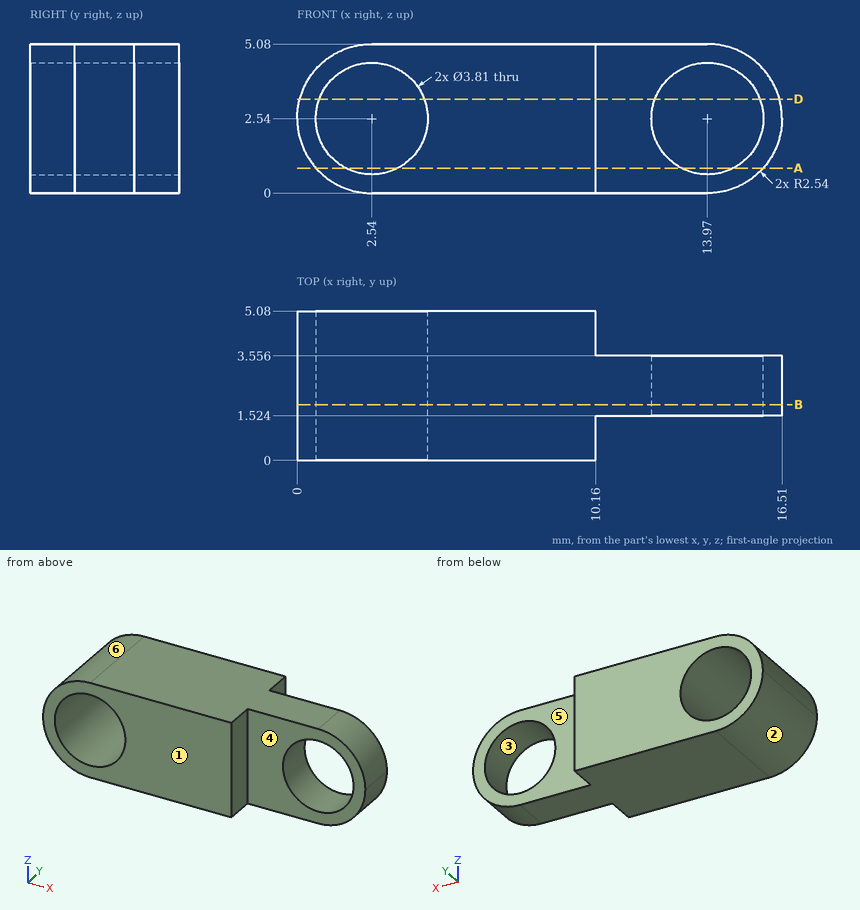
Geometry check sheet. Reference: drawing and pictorial views, mm from the part's lowest x, y, z. A direction names the side the tool comes from. Give positions to 0.01 mm unless a question says otherwise; leave off trailing zeros. Order: outer loops, then holes, each group sorted by start corner. A loop starts at its lowest first (then second) coordinate and runs counter-clockwise, first axis right, second up. Notation, with made-up numbers: M 20.25,70.25 L 62.25,70.25 A20 ccw 62.25,93.25 Z; hole C 53.25,36 d5. An arc over 180 degrees is marked long. Answer as a JSON object with one key per item and string values. Group by question number.
1) Cross-section at B-B (y = 1.9). Give the number of separate pieces and of enclosed holes in the cut face, then the cut area to 3 significant figures.
2) Depth check by flat-ended pin: pin 1 Ø0.8 at (y, z) = (0.5, 3) entering from +X; pin 2 Ø2.5 at (x, z) = (13.97, 2.54) entering from +Y; pin 3 Ø1 at (y, z) = (2, 1.5) entering from +X. Enter the tip coordinate at first touch or a pass-through.
3) Cross-section at A-A (z = 0.85). Enter the section's corners in (x, y).
4) Access from +Z, -Z, +X, -X, +Y, -Y to the whole of each face (thin tool, end or side, straight path). Record for the marked faces 4, 5 and 6.
5) Scan lines: line 1 along Z through (x, y) = (2.5, 1.8); line 2 along X through (y, z) = (2.65, 2.7); line 3 along X through (y, z) = (3.15, 1.8). Record each from-to range of solid material in increasing order. Write a range as [from, to].
6) Mould release check, pull along X, two halves, no side actions. Record for the marked faces 1, 2 and 3: released by +X, released by -X, zero draft, split by the parting line, or undercut.
7) Cross-section at D-D (z = 3.2). Enter the section's corners in (x, y), then the cut area to 3 significant figures.
Result sheet:
{
 "1": {"separate pieces": "1", "enclosed holes": "2", "area": "55.5 mm2"},
 "2": {"pin 1": "stops at x = 10.16", "pin 2": "passes through", "pin 3": "stops at x = 16.45"},
 "3": {"outline": "M 0.64,0 L 1.66,0 L 1.66,5.08 L 0.64,5.08 Z; M 3.42,0 L 10.16,0 L 10.16,1.52 L 13.09,1.52 L 13.09,3.56 L 10.16,3.56 L 10.16,5.08 L 3.42,5.08 Z; M 14.85,1.52 L 15.87,1.52 L 15.87,3.56 L 14.85,3.56 Z"},
 "4": {"face 4": "+Z, -Z, +X, -Y", "face 5": "+Z, -Z, +X, +Y", "face 6": "+Z, -X, +Y, -Y"},
 "5": {"line 1": "z = [0, 0.64], [4.44, 5.08]", "line 2": "x = [0.01, 0.64], [4.44, 12.07], [15.87, 16.5]", "line 3": "x = [0.11, 0.78], [4.3, 12.21], [15.73, 16.4]"},
 "6": {"face 1": "zero draft", "face 2": "released by -X", "face 3": "undercut"},
 "7": {"outline": "M 0.09,0 L 0.75,0 L 0.75,5.08 L 0.09,5.08 Z; M 4.33,0 L 10.16,0 L 10.16,1.52 L 12.18,1.52 L 12.18,3.56 L 10.16,3.56 L 10.16,5.08 L 4.33,5.08 Z; M 15.76,1.52 L 16.42,1.52 L 16.42,3.56 L 15.76,3.56 Z", "area": "38.5 mm2"}
}
